Here's how the part is built. I have some questions about the finished solid (model axes, mm). Coordinates: 2 decimals unless noted, no trailing zeros. Loops run counter-clockwise (first coordinate to the right, second up) from the corner with the lowest first, then second, coordinate; pieces in that order, holes last. Notation, with made-up numbers: (-17, 79.25) - (41, 79.25) arc R12 ccw to (41, 92.25) - close; hole circle Ø2 at (-4, 76). An arc over 180 degrees is marked (long way). Use a Markdown table: item, result.
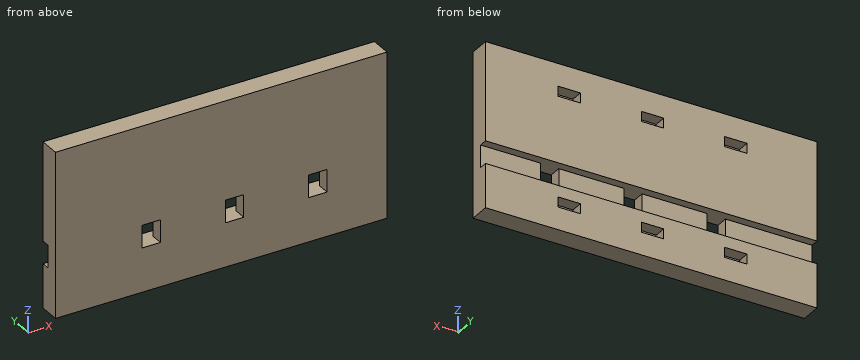
```python
from build123d import *

# Parameters (mm, degrees)
SKETCH1_W                     = 101.092
SKETCH1_H                     = 50.292
BOSS_EXTRUDE1_DEPTH           = 6.35
SKETCH2_W                     = 5.588
SKETCH2_H                     = 6.858
WIRE_HOLE_DEPTH               = 7.35
SKETCH3_W                     = 6.858
SKETCH3_H                     = 3.048
CUT_EXTRUDE2_DEPTH            = 3.81
LPATTERN1_COUNT               = 2
LPATTERN1_PITCH               = 25.4
LPATTERN1_COPY_1_SKETCH_W     = 6.858
LPATTERN1_COPY_1_SKETCH_H     = 3.048
LPATTERN1_COPY_1_DEPTH        = 3.81
LPATTERN1_COL_COUNT           = 2
LPATTERN1_COL_PITCH           = 25.4
LPATTERN1_COL_COPY_1_SKETCH_W = 6.858
LPATTERN1_COL_COPY_1_SKETCH_H = 3.048
LPATTERN1_COL_COPY_1_DEPTH    = 3.81
SKETCH4_W                     = 101.092
SKETCH4_H                     = 6.858
CUT_EXTRUDE3_DEPTH            = 2.54


with BuildPart() as part:
    # Sketch1 → Boss-Extrude1 (new body)
    with BuildSketch(Plane(origin=(0, 0, 0), x_dir=(1, 0, 0), z_dir=(0, 1, 0))):
        Rectangle(SKETCH1_W, SKETCH1_H)
    extrude(amount=BOSS_EXTRUDE1_DEPTH)

    # Sketch2 → Wire Hole (cut, through all)
    with BuildSketch(Plane(origin=(0, 6.35, 0), x_dir=(1, 0, 0), z_dir=(0, 1, 0))):
        with Locations((4.064, 8.322545685)):
            Rectangle(SKETCH2_W, SKETCH2_H)
    wire_hole = extrude(amount=-WIRE_HOLE_DEPTH, mode=Mode.SUBTRACT)

    # Sketch3 → Cut-Extrude2 (cut)
    with BuildSketch(Plane(origin=(0, 6.35, 0), x_dir=(1, 0, 0), z_dir=(0, 1, 0))):
        with Locations((-0.381, 16.764)):
            Rectangle(SKETCH3_W, SKETCH3_H)
    cut_extrude2 = extrude(amount=-CUT_EXTRUDE2_DEPTH, mode=Mode.SUBTRACT)

    # Mirror1: Cut-Extrude2 across plane
    add(cut_extrude2.mirror(Plane.XY), mode=Mode.SUBTRACT)

    # LPattern1: Wire Hole, Cut-Extrude2 ×2
    with Locations(*[(-i * LPATTERN1_PITCH, 0, 0) for i in range(1, LPATTERN1_COUNT)]):
        add(wire_hole, mode=Mode.SUBTRACT)
        add(cut_extrude2, mode=Mode.SUBTRACT)

    # LPattern1 copy 1 sketch → LPattern1 copy 1 (cut)
    with BuildSketch(Plane(origin=(-25.4, 6.35, 0), x_dir=(1, 0, 0), z_dir=(0, 1, 0))):
        with Locations((-0.381, -16.764)):
            Rectangle(LPATTERN1_COPY_1_SKETCH_W, LPATTERN1_COPY_1_SKETCH_H)
    extrude(amount=-LPATTERN1_COPY_1_DEPTH, mode=Mode.SUBTRACT)

    # LPattern1 col: Wire Hole, Cut-Extrude2 ×2
    with Locations(*[(i * LPATTERN1_COL_PITCH, 0, 0) for i in range(1, LPATTERN1_COL_COUNT)]):
        add(wire_hole, mode=Mode.SUBTRACT)
        add(cut_extrude2, mode=Mode.SUBTRACT)

    # LPattern1 col copy 1 sketch → LPattern1 col copy 1 (cut)
    with BuildSketch(Plane(origin=(25.4, 6.35, 0), x_dir=(1, 0, 0), z_dir=(0, 1, 0))):
        with Locations((-0.381, -16.764)):
            Rectangle(LPATTERN1_COL_COPY_1_SKETCH_W, LPATTERN1_COL_COPY_1_SKETCH_H)
    extrude(amount=-LPATTERN1_COL_COPY_1_DEPTH, mode=Mode.SUBTRACT)

    # Sketch4 → Cut-Extrude3 (cut)
    with BuildSketch(Plane(origin=(0, 6.35, 0), x_dir=(1, 0, 0), z_dir=(0, 1, 0))):
        with Locations((0, 8.322545685)):
            Rectangle(SKETCH4_W, SKETCH4_H)
    extrude(amount=-CUT_EXTRUDE3_DEPTH, mode=Mode.SUBTRACT)


solid = part.part
```
Q1. Please list where these lines run through material, in increasing order: L1, parallel to X at y = 4.75, z = 15.5; L2, parallel to Z at x = 3.5, y = 2.5; L3, parallel to X at y = 1.5, z = -5.5. Write a range as from..to.
Check values:
| item | result |
|---|---|
| L1 | -50.55..-29.21, -22.35..-3.81, 3.05..21.59, 28.45..50.55 |
| L2 | -25.15..-11.75, -4.89..25.15 |
| L3 | -50.55..-24.13, -18.54..1.27, 6.86..26.67, 32.26..50.55 |
Q2. Will this pin go through, and if not, where does the flat tip stop? P1, Ø2, axis at x = 14, z = -7.5, coming from the +Y side.
Check values:
| item | result |
|---|---|
| P1 | y = 3.81 |
Q3. I want a section at B-B, the plane z = -6. Write out the boundary of the cut face in (x, y).
Check values:
| item | result |
|---|---|
| outline | (-50.55, 0) - (-24.13, 0) - (-24.13, 3.81) - (-50.55, 3.81) - close; (-18.54, 0) - (1.27, 0) - (1.27, 3.81) - (-18.54, 3.81) - close; (6.86, 0) - (26.67, 0) - (26.67, 3.81) - (6.86, 3.81) - close; (32.26, 0) - (50.55, 0) - (50.55, 3.81) - (32.26, 3.81) - close |
Q4. I want a section at C-C, the plane x = -15. Write out the boundary of the cut face in (y, z).
Check values:
| item | result |
|---|---|
| outline | (0, -25.15) - (6.35, -25.15) - (6.35, -11.75) - (3.81, -11.75) - (3.81, -4.89) - (6.35, -4.89) - (6.35, 25.15) - (0, 25.15) - close |
Q5. I want a section at D-D, the plane x = 25.5. Write out the boundary of the cut face in (y, z), then the cut area to 3 significant figures.
Check values:
| item | result |
|---|---|
| outline | (0, -25.15) - (6.35, -25.15) - (6.35, -18.29) - (2.54, -18.29) - (2.54, -15.24) - (6.35, -15.24) - (6.35, -11.75) - (3.81, -11.75) - (3.81, -4.89) - (6.35, -4.89) - (6.35, 15.24) - (2.54, 15.24) - (2.54, 18.29) - (6.35, 18.29) - (6.35, 25.15) - (0, 25.15) - close |
| area | 279 mm^2 |
Q6. I want a section at A-A, the plane y = 1.25. Write out the boundary of the cut face in (x, z), then the cut area to 3 significant figures.
Check values:
| item | result |
|---|---|
| outline | (-50.55, -25.15) - (50.55, -25.15) - (50.55, 25.15) - (-50.55, 25.15) - close; hole (-24.13, -11.75) - (-18.54, -11.75) - (-18.54, -4.89) - (-24.13, -4.89) - close; hole (1.27, -11.75) - (6.86, -11.75) - (6.86, -4.89) - (1.27, -4.89) - close; hole (26.67, -11.75) - (32.26, -11.75) - (32.26, -4.89) - (26.67, -4.89) - close |
| area | 4,970 mm^2 |
